```python
from build123d import *

# Parameters (mm, degrees)
SKETCH1_W           = 4.7625
SKETCH1_H           = 9
BOSS_EXTRUDE1_DEPTH = 1.984375
FILLET1_R           = 0.5
FILLET2_R           = 0.5


with BuildPart() as part:
    # Sketch1 → Boss-Extrude1 (new body)
    with BuildSketch(Plane.XY):
        with Locations((2.38125, 4.5)):
            Rectangle(SKETCH1_W, SKETCH1_H)
    extrude(amount=BOSS_EXTRUDE1_DEPTH)

    # Fillet1
    fillet1_edges = [part.edges().sort_by_distance(p)[0] for p in [
        (0, 9, 0.9921875),
        (4.7625, 9, 0.9921875),
    ]]
    fillet(fillet1_edges, radius=FILLET1_R)

    # Fillet2
    fillet2_edges = [part.edges().sort_by_distance(p)[0] for p in [
        (4.7625, 0, 0.9921875),
        (0, 0, 0.9921875),
    ]]
    fillet(fillet2_edges, radius=FILLET2_R)


solid = part.part
```
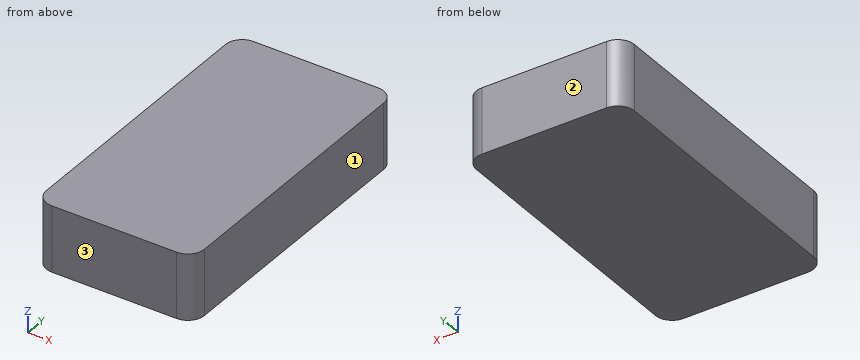
The model under review builds one solid part; all positions refer to its coordinate system, in mm. Face numbers are marked on the shaded views. Give positions to 0.01 mm unless a question says otherwise; leave off trailing zeros. Answer as a JSON object with one key per item and string values.
Q1. To check wall thickness, follow line 1 along Y through (x, z) = (4.3, 1.25); line 2 along Y through (x, z) = (4.5, 0.75); line 3 along X through (y, z) = (8.75, 1.15). State the ranges of each line that lie inside material, in increasing order.
Worked out:
{"line 1": "y = 0 to 9", "line 2": "y = 0.06 to 8.94", "line 3": "x = 0.07 to 4.7"}
Q2. Mouldability with a two-part tool opening along Y and no side actions: class the marked faces 1, 2 and 3 as +Y half, -Y half, draft (parallel to the pull), parting line (faces both ways), or undercut.
Worked out:
{"face 1": "draft", "face 2": "+Y half", "face 3": "-Y half"}
Q3. Insertion check: pin 1 (2 mm diameter, centred on x = 0.5, y = 6, fed in from -Z). The pin has a flat end and moves straight along its axis. Give the tip position at first contact, or say it passes through.
Worked out:
{"pin 1": "stops at z = 0"}
